```python
from build123d import *

# Parameters (mm, degrees)
SKETCH1_W           = 70
SKETCH1_H           = 76.2
SKETCH1_R           = 1.75
SKETCH1_R_2         = 12
BOSS_EXTRUDE1_DEPTH = 6.35


with BuildPart() as part:
    # Sketch1 → Boss-Extrude1 (new body)
    with BuildSketch(Plane.XY):
        Rectangle(SKETCH1_W, SKETCH1_H)
        with Locations((0, 28.1)):
            Circle(SKETCH1_R, mode=Mode.SUBTRACT)
        with Locations((17.320508076, -1.9)):
            Circle(SKETCH1_R, mode=Mode.SUBTRACT)
        with Locations((-17.320508076, -1.9)):
            Circle(SKETCH1_R, mode=Mode.SUBTRACT)
        with Locations((0, 8.1)):
            Circle(SKETCH1_R_2, mode=Mode.SUBTRACT)
        with BuildLine():
            Line((-32.05, 25.6), (-32.05, 30.6))
            ThreePointArc((-32.05, 30.6), (-30, 32.65), (-27.95, 30.6))
            Line((-27.95, 30.6), (-27.95, 25.6))
            ThreePointArc((-27.95, 25.6), (-30, 23.55), (-32.05, 25.6))
        make_face(mode=Mode.SUBTRACT)
        with BuildLine():
            Line((32.05, 25.6), (32.05, 30.6))
            ThreePointArc((32.05, 30.6), (30, 32.65), (27.95, 30.6))
            Line((27.95, 30.6), (27.95, 25.6))
            ThreePointArc((27.95, 25.6), (30, 23.55), (32.05, 25.6))
        make_face(mode=Mode.SUBTRACT)
        with BuildLine():
            Line((-32.05, -25.6), (-32.05, -30.6))
            ThreePointArc((-32.05, -30.6), (-30, -32.65), (-27.95, -30.6))
            Line((-27.95, -30.6), (-27.95, -25.6))
            ThreePointArc((-27.95, -25.6), (-30, -23.55), (-32.05, -25.6))
        make_face(mode=Mode.SUBTRACT)
        with BuildLine():
            Line((32.05, -25.6), (32.05, -30.6))
            ThreePointArc((32.05, -30.6), (30, -32.65), (27.95, -30.6))
            Line((27.95, -30.6), (27.95, -25.6))
            ThreePointArc((27.95, -25.6), (30, -23.55), (32.05, -25.6))
        make_face(mode=Mode.SUBTRACT)
    extrude(amount=BOSS_EXTRUDE1_DEPTH)


solid = part.part
```
Check sheet for the modelled part. Datum: model origin and axes. Units: mm. A direction names the side the tool comes from. Coordinates: 2 decimals unless noted, no trailing zeros. Write each loop counter-clockwise with the first axis right and the second up, starting at its lowest first coordinate (ties: lowest second). Pieces come first, ordered by that corner, then holes. Notation, with made-up numbers: (68, -2.75) -> (98, -2.75) arc R11 ccw to (98, 14.25) -> close; hole circle Ø2 at (5.5, 42.5). An arc over 180 degrees is marked (long way). Use a Markdown table: item, result.
1. Sectioned sample at B-B (y = 8.1). Enter the section's corners in (x, z).
Reported:
| item | result |
|---|---|
| outline | (-35, 0) -> (-12, 0) -> (-12, 6.35) -> (-35, 6.35) -> close; (12, 0) -> (35, 0) -> (35, 6.35) -> (12, 6.35) -> close |
2. Sectioned sample at D-D (x = 8.5). Enter the section's corners in (y, z).
Reported:
| item | result |
|---|---|
| outline | (-38.1, 0) -> (-0.37, 0) -> (-0.37, 6.35) -> (-38.1, 6.35) -> close; (16.57, 0) -> (38.1, 0) -> (38.1, 6.35) -> (16.57, 6.35) -> close |
3. Tool access check on faces 1 (the flat face through (0, -8, 6.35)), 2 (the flat face through (27.95, -28, 3)). Record the directions out of +Z, -Z, +X, -X, +Y, -Y that give a thin tool (end or side, any length) a straight path to the whole face; none if there is none.
Reported:
| item | result |
|---|---|
| face 1 | +Z, +X, -X, +Y, -Y |
| face 2 | +Z, -Z |
4. Release check for a two-part mould opening along Y. For faces 3 (the flat face through (0, -38.1, 3)), 4 (the cylindrical face through (-19.07, -1.82, 3.13)), 5 (the flat face through (0, -8, 0)), 6 (the flat face through (27.95, 28, 3)) record: pulls with the +Y half, pulls with the -Y half, needs draft (parallel to the pull), parting line crosses it, or undercut.
Reported:
| item | result |
|---|---|
| face 3 | pulls with the -Y half |
| face 4 | undercut |
| face 5 | needs draft |
| face 6 | undercut |
5. Sectioned sample at C-C (z = 4.5). Give the number of separate pieces and of enclosed holes in the cut face, plus the area to 3 significant figures.
Reported:
| item | result |
|---|---|
| separate pieces | 1 |
| enclosed holes | 8 |
| area | 4,720 mm2 |
6. Go/stop test with flat-tipped pins: pin 1 Ø10 at (x, y) = (5.5, -17.5) entering from -Z; pin 2 Ø3 at (x, y) = (0, 28.1) entering from +Z. Record where each tip stops, or that it passes through.
Reported:
| item | result |
|---|---|
| pin 1 | stops at z = 0 |
| pin 2 | passes through |
7. Scan lines: line 1 along X through (y, z) = (-25.5, 5); line 2 along Y through (x, z) = (28.5, 4.25); line 3 along X through (y, z) = (0.5, 3.5). Record each from-to range of solid material in increasing order.
Reported:
| item | result |
|---|---|
| line 1 | x = -35 to -32.05, -27.95 to 27.95, 32.05 to 35 |
| line 2 | y = -38.1 to -32, -24.2 to 24.2, 32 to 38.1 |
| line 3 | x = -35 to -9.29, 9.29 to 35 |
8. Sectioned sample at A-A (y = 28.1). Enter the section's corners in (x, z), plus the area to 3 significant figures.
Reported:
| item | result |
|---|---|
| outline | (-35, 0) -> (-32.05, 0) -> (-32.05, 6.35) -> (-35, 6.35) -> close; (-27.95, 0) -> (-1.75, 0) -> (-1.75, 6.35) -> (-27.95, 6.35) -> close; (1.75, 0) -> (27.95, 0) -> (27.95, 6.35) -> (1.75, 6.35) -> close; (32.05, 0) -> (35, 0) -> (35, 6.35) -> (32.05, 6.35) -> close |
| area | 370 mm2 |
